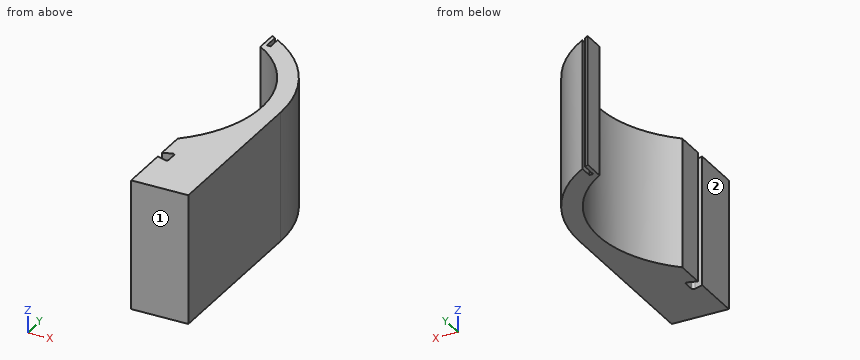
from build123d import *

# Parameters (mm, degrees)
INNER_RING_RIGHT_SIDE_DEPTH = 170


with BuildPart() as part:
    # Sketch2 → Inner Ring - Right Side (new body)
    with BuildSketch(Plane.XY):
        with BuildLine():
            Line((100, -111.803398875), (100, -150))
            Line((100, -150), (111.709430585, -146.096856472))
            ThreePointArc((111.709430585, -146.096856472), (113.961775712, -146.440459254), (115, -148.468564717))
            Line((115, -148.468564717), (115, -161.531435283))
            ThreePointArc((115, -161.531435283), (113.961775712, -163.559540746), (111.709430585, -163.903143528))
            Line((111.709430585, -163.903143528), (100, -160))
            Line((100, -160), (100, -225))
            Line((100, -225), (175, -225))
            Line((175, -225), (175, 0))
            ThreePointArc((175, 0), (152.274423328, 86.240941553), (90, 150.083310198))
            Line((90, 150.083310198), (90, 132.970585408))
            Line((90, 132.970585408), (85, 132.970585408))
            Line((85, 132.970585408), (85, 152.970585408))
            ThreePointArc((85, 152.970585408), (82.510826874, 154.327455265), (80, 155.643824163))
            Line((80, 155.643824163), (80, 126.885775404))
            ThreePointArc((80, 126.885775404), (149.476186998, 12.524756303), (100, -111.803398875))
        make_face()
    extrude(amount=INNER_RING_RIGHT_SIDE_DEPTH)


solid = part.part
For this review, take the finished solid that the model builds, in its own axes (mm). Face numbers are marked on the shaded views. A direction names the side the tool comes from. Give positions to 0.01 mm unless a question says otherwise; leave off trailing zeros. Loops run counter-clockwise (first coordinate to the right, second up) from the corner with the lowest first, then second, coordinate; pieces in that order, holes last. Notation, with made-up numbers: M 14,66 L 64,66 A8 cw 64,72 Z; hole C 62.25,-13.5 d2. An arc over 180 degrees is marked long. Answer as a JSON object with one key per item and string values. Group by question number.
Q1. Add section B-B on x = 138.5. Give the boundary of the cut face in (y, z).
Q2. Add section A-A on z = 88. Give the boundary of the cut face in (x, y).
Q3. For probe 1 along Y at (x, z) = (107, 25.5); probe 2 along X at (y, z) = (-152, 156.5); probe 3 along Y at (x, z) = (133.5, 14), list the stretches that pass through material, from the lowest coordinate up. Write a range as [from, to].
Q4. Tool access review of the marked faces 1 and 2: name each direction out of +Z, -Z, +X, -X, +Y, -Y from which nothing blocks a thin tool from reaching the whole face with its end or side.
Q5. Insertion check: P1, Ø22, axis at y = 143.5, z = 102.5, coming from the +X side; P2, Ø19, axis at y = -122.5, z = 90, coming from the -X side; P3, Ø2, axis at x = 119, z = 75.5, coming from the +Y side. Each pin has a flat end and moves straight along its axis. Give the tip position at first contact, or say it passes through.
Q6. Add section D-D on y = -184. Give the boundary of the cut face in (x, z).
Q7. Add section C-C on x = 106.5. Give the boundary of the cut face in (y, z), and give its area (3 significant figures).
Checked values:
{
 "1": {"outline": "M -225,0 L -57.6,0 L -57.6,170 L -225,170 Z; M 57.6,0 L 106.97,0 L 106.97,170 L 57.6,170 Z"},
 "2": {"outline": "M 80,126.89 A150 cw 100,-111.8 L 100,-150 L 111.71,-146.1 A2.5 cw 115,-148.47 L 115,-161.53 A2.5 cw 111.71,-163.9 L 100,-160 L 100,-225 L 175,-225 L 175,0 A175 ccw 90,150.08 L 90,132.97 L 85,132.97 L 85,152.97 A175 ccw 80,155.64 Z"},
 "3": {"probe 1": "[-225, -162.33], [-147.67, -105.12], [105.12, 138.48]", "probe 2": "[115, 175]", "probe 3": "[-225, -68.39], [68.39, 113.15]"},
 "4": {"face 1": "+Z, -Z, +X, -X, -Y", "face 2": "+Z, -Z, -X, -Y"},
 "5": {"P1": "x = 114.32", "P2": "x = 100", "P3": "y = 129.23"},
 "6": {"outline": "M 100,0 L 175,0 L 175,170 L 100,170 Z"},
 "7": {"outline": "M -225,0 L -162.17,0 L -162.17,170 L -225,170 Z; M -147.83,0 L -105.63,0 L -105.63,170 L -147.83,170 Z; M 105.63,0 L 138.86,0 L 138.86,170 L 105.63,170 Z", "area": "23,500 mm²"}
}
